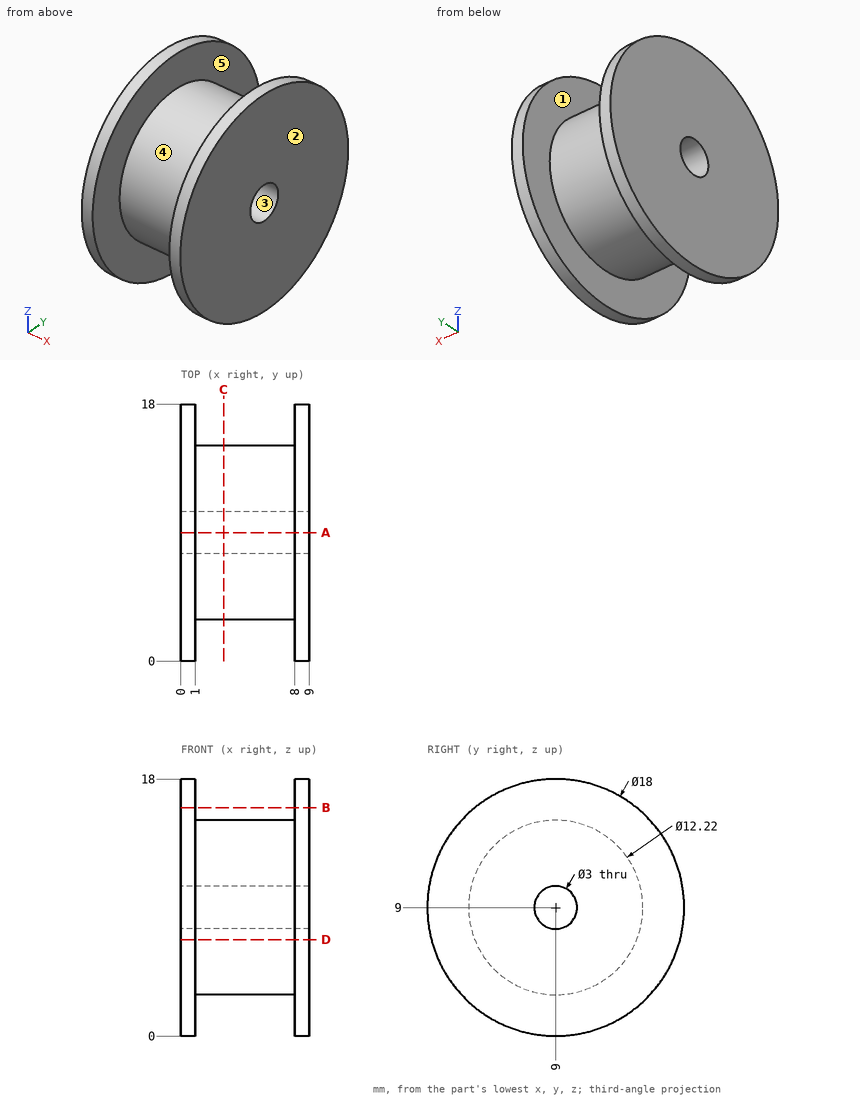
Could you check a few things on this drawing? It's one solid part, dimensions in mm from its lowest x, y, z. A direction names the side the tool comes from. Coordinates: 2 decimals unless noted, no trailing zeros. Order: outer loops, then holes, each group sorted by start corner. A loop starts at its lowest first (then second) coordinate and runs counter-clockwise, first axis right, second up. Notation, with made-up numbers: M 79.5,-37.5 L 121.5,-37.5 A21 ccw 121.5,-14.5 Z; hole C -28.75,30.5 d5. An arc over 180 degrees is marked long. Answer as a JSON object with one key per item and string values. Group by question number.
(1) Suppose I cut it at D-D, the plane z = 6.75. Please give me the cut outline in (x, y), then the cut area to 3 significant figures.
(2) For pin 1 (1.5 mm diameter, centred on x = 3.5, z = 12, fed in from +Y); pin 2 (4 mm diameter, centred on x = 1, y = 5, fed in from +Z), each with a flat end and sliding along its axis, tell me the tip position at first contact or that it passes through.
(3) I need wall thicknesses on probe 1 along X at (y, z) = (12.5, 17.25); probe 2 along Z at (x, y) = (3.75, 9); probe 3 along Z at (x, y) = (5.25, 8). Which ranges of each line are inside material? Lowest first, please.
(4) Which directions (+Z, -Z, +X, -X, +Y, -Y) give clear straight access to the entire face, cutting with the end or side of a thin tool? Please do the marked faces 1 and 2.
(5) Suppose I cut it at C-C, the plane x = 3. Please give me the cut outline in (y, z).
(6) Suppose I cut it at B-B, the plane z = 16. Please give me the cut outline in (x, y).
(7) If we mould it in two halves opening along Y, with no side actions, what happens to the marked faces 3, 4 and 5? For each: released by +Y, released by -Y, zero draft, split by the parting line, or undercut.
(8) Suppose I cut it at A-A, the plane y = 9. Please give me the cut outline in (x, z).
Values found:
{
 "1": {"outline": "M 0,0.29 L 1,0.29 L 1,3.32 L 8,3.32 L 8,0.29 L 9,0.29 L 9,17.71 L 8,17.71 L 8,14.68 L 1,14.68 L 1,17.71 L 0,17.71 Z", "area": "114 mm^2"},
 "2": {"pin 1": "stops at y = 14.68", "pin 2": "stops at z = 17.77"},
 "3": {"probe 1": "x = 0 to 1, 8 to 9", "probe 2": "z = 2.89 to 7.5, 10.5 to 15.11", "probe 3": "z = 2.97 to 7.88, 10.12 to 15.03"},
 "4": {"face 1": "none", "face 2": "+Z, -Z, +X, +Y, -Y"},
 "5": {"outline": "C 9,9 d12.22; hole C 9,9 d3"},
 "6": {"outline": "M 0,3.34 L 1,3.34 L 1,14.66 L 0,14.66 Z; M 8,3.34 L 9,3.34 L 9,14.66 L 8,14.66 Z"},
 "7": {"face 3": "undercut", "face 4": "split by the parting line", "face 5": "zero draft"},
 "8": {"outline": "M 0,0 L 1,0 L 1,2.89 L 8,2.89 L 8,0 L 9,0 L 9,7.5 L 0,7.5 Z; M 0,10.5 L 9,10.5 L 9,18 L 8,18 L 8,15.11 L 1,15.11 L 1,18 L 0,18 Z"}
}
